from build123d import *

# Parameters (mm, degrees)
F2_DEPTH      = 9.7
F2_DEPTH_BACK = 21.7
F0_R          = 8.875
F3_DEPTH      = 25
F3_DEPTH_BACK = 25
F5_DEPTH      = 25
F5_DEPTH_BACK = 25


with BuildPart() as f2:
    # F1 (on Top) → F2 (new body, two sides)
    with BuildSketch(Plane.XY) as f2_sk:
        with BuildLine():
            ThreePointArc((11.0648144764, -3.4107860847), (11.4494203432, -1.7246318209), (11.5785828629, 0))
            ThreePointArc((11.5785828629, 0), (11.3390271612, 2.3430843246), (10.6302726566, 4.5892139153))
            ThreePointArc((10.6302726566, 4.5892139153), (0, 5.2871789927), (-10.6302726566, 4.5892139153))
            ThreePointArc((-10.6302726566, 4.5892139153), (-11.5615397516, 0.6279965655), (-11.0648144764, -3.4107860847))
            ThreePointArc((-11.0648144764, -3.4107860847), (0, -4.3353080989), (11.0648144764, -3.4107860847))
        make_face()
    extrude(amount=-F2_DEPTH)
    extrude(f2_sk.sketch, amount=F2_DEPTH_BACK)

    # F0 (on Front) → F3 (cut, two sides)
    with BuildSketch(Plane.XZ) as f3_sk:
        Circle(F0_R)
    extrude(amount=-F3_DEPTH, mode=Mode.SUBTRACT)
    extrude(f3_sk.sketch, amount=F3_DEPTH_BACK, mode=Mode.SUBTRACT)

    # F4 (on Right) → F5 (cut, two sides)
    with BuildSketch(Plane.YZ) as f5_sk:
        with BuildLine():
            ThreePointArc((0, 30.6800138205), (3.7581649162, 5.252439566), (6.1427378096, -20.3405115753))
            ThreePointArc((6.1427378096, -20.3405115753), (0.1999286469, 33.1697739229), (-5.7428805158, -20.3405115753))
            ThreePointArc((-5.7428805158, -20.3405115753), (-2.2708328186, 5.1021466294), (0, 30.6800138205))
        make_face()
    extrude(amount=-F5_DEPTH, mode=Mode.SUBTRACT)
    extrude(f5_sk.sketch, amount=F5_DEPTH_BACK, mode=Mode.SUBTRACT)


solid = f2.part
Model file for the job. Use its own axes, mm. Give positions to 0.01 mm unless a question says otherwise; leave off trailing zeros. Order: outer loops, then holes, each group sorted by start corner. A loop starts at its lowest first (then second) coordinate and runs counter-clockwise, first axis right, second up. Notation, with made-up numbers: M -25,29 L 15,29 A18 cw 15,48 Z; hole C 31,76.5 d9. An arc over 180 degrees is marked long. Put each result on its own line as item: value. Start each with the question number.
(1) Band-saw the part on C-C on y = -2. Give the cut face in (x, z) (3 decimals), then the cut area to 3 significant figures.
(2) Pull direction X, two halves, no side cores. Call faces 1 (the face through (-1.924, 0.545, -8.664)), 2 (the face through (0, 1, -9.7)), 3 (the face through (11.565, 0.571, 2.291)): released by +X, released by -X, zero draft, split by the parting line, or undercut.
(3) Band-saw the part on D-D on x = -5.5. Give the cut face in (y, z).
(4) Drill centre lines: L1, parallel to X at y = -0.75, z = 0 (3 decimals); L2, parallel to Z at x = 0, y = 1.25 (3 decimals); L3, parallel to X at y = -2, z = 0 (3 decimals). Where is each one in solid material? Low to high. Write a range as [from, to].
(5) Band-saw the part on B-B on z = 0. Give the cut face in (x, y) (3 decimals).
(6) Band-saw the part on A-A on x = -8. Give the cut face in (y, z).
(7) Pin check, flat tips, straight feed: pin 1 Ø8 at (x, z) = (2.5, 17) entering from -Y; pin 2 Ø1.5 at (x, z) = (1.5, 12.5) entering from -Y; pin 3 Ø2 at (y, z) = (3, -3) entering from -X. Stop position of each tip, or through.
Results below:
1. outline: M -11.405,-9.7 L 11.405,-9.7 L 11.405,7.558 L 4.652,7.558 A8.875 cw long -4.652,7.558 L -11.405,7.558 Z
1. area: 154 mm2
2. face 1: undercut
2. face 2: zero draft
2. face 3: released by +X
3. outline: M -4.11,-9.7 L 5.1,-9.7 L 5.1,-7.3 A477.54 ccw 5.07,-6.97 L -3.77,-6.97 A545.49 cw -4.11,-9.46 Z; M -2.06,6.97 L 3.55,6.97 A477.54 ccw 1.49,21.7 L -0.66,21.7 A545.49 cw Z
4. L1: x = [-11.554, -8.875], [8.875, 11.554]
4. L2: z = [-9.7, -8.875], [8.875, 21.7]
4. L3: x = [-11.405, -8.875], [8.875, 11.405]
5. outline: M -11.217,-2.869 L -8.875,-2.869 L -8.875,4.361 L -10.726,4.361 A11.579 ccw Z; M 8.875,-2.869 L 11.217,-2.869 A11.579 ccw 10.726,4.361 L 8.875,4.361 Z
6. outline: M -3.85,-9.7 L 4.89,-9.7 L 4.89,-5.12 A477.54 ccw 4.76,-3.84 L -3.35,-3.84 A545.49 cw -3.85,-7.61 Z; M -2.41,3.84 L 3.93,3.84 A477.54 ccw 1.49,21.7 L -0.66,21.7 A545.49 cw Z
7. pin 1: stops at y = -1.44
7. pin 2: stops at y = -1.56
7. pin 3: stops at x = -11.4
